Autodesk Inventor part; units mm, degrees
ref_plane "YZ Plane" through (0, 0, 0) normal (1, 0, 0) x (0, 1, 0)
ref_plane "XZ Plane" through (0, 0, 0) normal (0, 1, 0) x (-1, 0, 0)
ref_plane "XY Plane" through (0, 0, 0) normal (0, 0, 1) x (1, 0, 0)
sketch "Sketch1" plane through (0, 0, 0) normal (0, 0, 1) x (1, 0, 0)
  line L0 (-490, 63) -> (490, 63)
  line L1 (490, 63) -> (490, 0)
  line L2 (490, 0) -> (-490, 0)
  line L3 (-490, 0) -> (-490, 63)
  point P0 (0, 0)
  point P1 (0, 0)
  dimension "d0" = 980
  dimension "d1" = 63
extrude "Plate1" add sketch "Sketch1" along normal blind 2
sketch "Sketch2" plane through (490, -2, 0) normal (0, 1, 0) x (-1, 0, 0)
  line L0 (980, 0) -> (0, 0)
  line L1 (0, 0) -> (0, 20)
  line L2 (0, 20) -> (980, 20)
  line L3 (980, 20) -> (980, 0)
edge flange "Flange1" height 20 angle 90 thickness 2 bend radius 2.75 thickness toward (0, 1, 0) relief round relief width 2 relief depth 1 edges at (0, 0, 2) wall of the first edge with corners at (-490, -2, 0) (490, -2, 0) (490, -2, 20) (-490, -2, 20)
bend "Bend1"
corner "Corner1"
sketch "Sketch5" plane through (0, 0, 0) normal (0, 0, -1) x (-1, 0, 0)
  line L0 (490, 63) -> (-490, 63)
  line L1 (490, -2) -> (-490, -2)
  circle A0 centre (0, 63) radius 17.5
  line L2 (243.95, 63) -> (246.05, 63)
  line L3 (246.05, 63) -> (246.05, 26)
  line L4 (246.05, 26) -> (243.95, 26)
  line L5 (243.95, 26) -> (243.95, 63)
  line L6 (-243.95, 63) -> (-246.05, 63)
  line L7 (-246.05, 63) -> (-246.05, 26)
  line L8 (-246.05, 26) -> (-243.95, 26)
  line L9 (-243.95, 26) -> (-243.95, 63)
  line L10 (0, 63) -> (0, -2) construction
  point P0 (0, 0)
  point P1 (-490, -2)
  point P2 (245, 26)
  point P3 (-245, 26)
  point P4 (246.05, 63)
  point P5 (-17.5, 63)
  point P6 (17.5, 63)
  point P7 (-246.05, 63)
  dimension "d45" = 35
  dimension "d48" = 2.1
  dimension "d49" = 490
  dimension "d51" = 28
  dimension "d52" = 37
extrude "Extrusion1" cut sketch "Sketch5" against normal through all contours L3 L4 L5 L0 | L9 L8 L7 L0 | A0 L0 picked at (-2.238, 56.1497)
sketch "Sketch9" plane through (0, 0, 2) normal (0, 0, 1) x (1, 0, 0)
  line L0 (485.6141, 29.596) -> (485.6141, 17.596) construction
  line L1 (485.6141, 17.596) -> (285.6141, 17.596) construction
  line L2 (285.6141, 17.596) -> (285.6141, 29.596) construction
  line L3 (285.6141, 29.596) -> (485.6141, 29.596) construction
  line L4 (-490, 63) -> (490, 63)
  point P0 (0, 0)
  point P1 (1.05, 68)
  point P2 (490, 63)
  dimension "d40" = 200
  dimension "d41" = 12
mark "Mark2"
equation "\"d2\" = Thickness"
equation "\"d3\" = BendReliefWidth"
equation "\"d4\" = BendReliefDepth"
equation "\"d5\" = MinimumRemnant"
equation "\"d6\" = TransitionRadius"
equation "\"d9\" = BendRadius"
equation "\"d10\" = CornerReliefSize"
equation "\"d11\" = GapSize"
equation "\"d12\" = JacobiRadiusSize"
equation "\"BendReliefWidth\" = Thickness"
equation "\"BendReliefDepth\" = 0.5 * Thickness"
equation "\"CornerReliefSize\" = 4 * Thickness"
equation "\"MinimumRemnant\" = 2 * Thickness"
equation "\"TransitionRadius\" = BendRadius"
equation "\"JacobiRadiusSize\" = BendRadius"
equation "\"GapSize\" = Thickness"
properties part number "MSC 322 STRINGER BOARD  #" material "Stainless Steel"
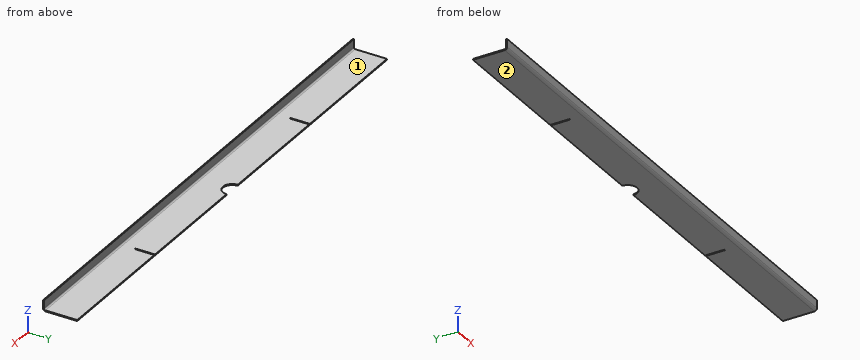
CAD build for the part. Positions are in the model's coordinates, mm. Face numbers are marked on the shaded views. A direction names the side the tool comes from. Give positions to 0.01 mm unless a question says otherwise; leave off trailing zeros. Order: outer loops, then holes, each group sorted by start corner. A loop starts at its lowest first (then second) coordinate and runs counter-clockwise, first axis right, second up.
(1) Flat gauge pins, fed straight in: pin 1 (1.5 mm diameter, centred on x = -124, y = 56, fed in from +Z); pin 2 (12 mm diameter, centred on x = -198.5, z = 15, fed in from +Y); pin 3 (10 mm diameter, centred on y = 35, z = 11, fed in from -X); pin 4 (1.6 mm diameter, centred on x = -245, z = 0.5, fed in from +Y). Where does each tip first touch, or does it go through?
(2) Saw through at A-A, the plane x = -294.5. Give the cut face in (y, z), then the cut area to 3 significant figures.
(3) Tool access for the marked faces 1 and 2: list every direction of +Z, -Z, +X, -X, +Y, -Y with a clear straight run to the whole face (end or side of a thin tool).
(4) Drill centre lines: L1, parallel to Z at x = -248.5, y = 50.5; L2, parallel to Y at x = -368, z = 4; L3, parallel to Y at x = -74, z = 13.25. Where is each one in solid material? Low to high.
(5) Saw through at B-B, the plane z = 14.5. Give the cut face in (x, y).
(6) Saw through at C-C, the plane x = 0. Give the cut face in (y, z).
Results found:
1. pin 1: stops at z = 2
1. pin 2: stops at y = 0
1. pin 3: passes through
1. pin 4: stops at y = 26
2. outline: (-2, 4.75) arc R4.75 ccw to (2.75, 0) - (63, 0) - (63, 2) - (2.75, 2) arc R2.75 cw to (0, 4.75) - (0, 20) - (-2, 20) - close
2. area: 163 mm2
3. face 1: +Z, +X, -X, +Y
3. face 2: -Z, +X, -X, +Y, -Y
4. L1: z = 0 to 2
4. L2: y = -1.94 to 0.1
4. L3: y = -2 to 0
5. outline: (-490, -2) - (490, -2) - (490, 0) - (-490, 0) - close
6. outline: (-2, 4.75) arc R4.75 ccw to (2.75, 0) - (45.5, 0) - (45.5, 2) - (2.75, 2) arc R2.75 cw to (0, 4.75) - (0, 20) - (-2, 20) - close
